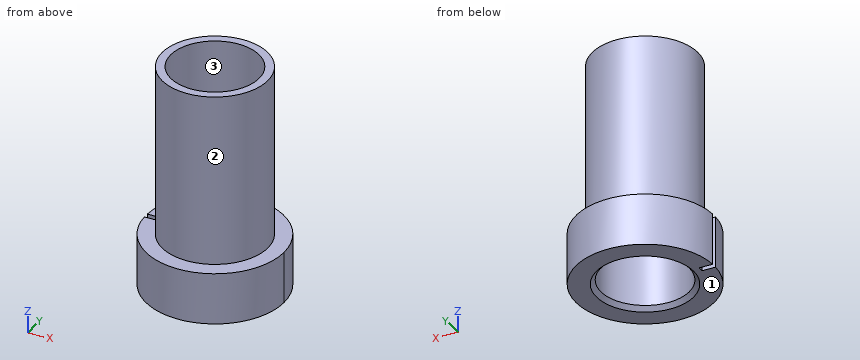
Autodesk Fusion 360 part; units mm, degrees
sketch "Sketch1" plane through (0, 0, 0) normal (0, 0, 1) x (1, 0, 0) in component "SpoolBottom"
  circle A0 centre (0, 0) radius 6.35
  dimension "d49" = 12.7
extrude "Extrude1" add sketch "Sketch1" along normal blind 4.7625 in component "SpoolBottom"
sketch "Sketch2" plane through (0, 0, 4.7625) normal (0, 0, 1) x (-1, 0, 0) in component "SpoolBottom"
  circle A0 centre (0, 0) radius 6.35
  circle A1 centre (0, 0) radius 4.8617
  dimension "d52" = 9.7234
extrude "Extrude2" add sketch "Sketch2" along normal blind 15.875 contours A1 in component "SpoolBottom"
sketch "Sketch3" plane through (0, 0, 20.6375) normal (0, 0, 1) x (-1, 0, 0) in component "SpoolBottom"
  circle A0 centre (0, 0) radius 4.8617
  circle A1 centre (0, 0) radius 4.068
  dimension "d55" = 8.1359
extrude "Extrude3" cut sketch "Sketch3" against normal blind 21.59 contours A1 in component "SpoolBottom"
chamfer "Chamfer1" distance 0.3969 angle 45 1 edges at (3.7927, 1.471, 0) in component "SpoolBottom"
sketch "Sketch4" plane through (0, 0, 4.7625) normal (0, 0, 1) x (-1, 0, 0) in component "SpoolBottom"
  circle A0 centre (0, 0) radius 4.8617
  circle A1 centre (0, 0) radius 6.35
  line L0 (5.0818, 0.2586) -> (6.5041, 0.2586)
  line L1 (6.5041, 0.2586) -> (6.5041, -0.2527)
  line L2 (6.5041, -0.2527) -> (5.0818, -0.2527)
  line L3 (5.0818, -0.2527) -> (5.0818, 0.2586)
extrude "Extrude4" cut sketch "Sketch4" against normal blind 4.826 contours A1 L0 L2 L3 picked at (5.5046, 0.002) in component "SpoolBottom"
component "SpoolBottom" placed x (1, 0, 0) y (0, 1, 0) z (0, 0, 1) at (0, 0, 0)
equation "d50 = ( 3 / 16 ) * 1 in"
equation "d52 = ( 5 / 16 ) * 1 in + ( 1 / 128 ) * 1 in + ( 2 / 32 ) * 1 in"
equation "d53 = ( 5 / 8 ) * 1 in"
equation "d55 = ( 5 / 16 ) * 1 in + ( 1 / 128 ) * 1 in"
equation "d58 = ( 1 / 64 ) * 1 in"
Source: CAD feature listing. Evaluate the final solid. Frame: model axes, mm. Face numbers are marked on the shaded views. Give positions to 0.01 mm unless a question says otherwise; leave off trailing zeros. Write each loop counter-clockwise with the first axis right and the second up, starting at its lowest first coordinate (ties: lowest second). Pieces come first, ordered by that corner, then holes.
1. Material intervals for line 1 along X through (y, z) = (0, 5); line 2 along Y through (x, z) = (0, 4.5), sorted ascending.
2. Pull-direction query (X, two-part tool) for the marked faces 1, 2 and 3; classes: +X half, -X half, draft (parallel to the pull), parting line (faces both ways), or undercut.
3. Section query A-A (x = 0). Return the cut outline in (y, z), then the cut area to 3 significant figures.
4. First-contact query: pin 1 (4 mm diameter, centred on x = 0.5, y = -0.5, fed in from +Z); pin 2 (4 mm diameter, centred on x = 3.5, z = 17.5, fed in from -Y); pin 3 (1 mm diameter, centred on x = -5.5, z = 3, fed in from -Y); pin 4 (1 mm diameter, centred on y = 3, z = 15.5, fed in from -X). Flat tips, straight axial feed; report the tip coordinate or a pass-through.
5. Section query B-B (z = 5). Return the cut outline in (x, y).
Output values:
1. line 1: x = -4.86 to -4.07, 4.07 to 4.86
1. line 2: y = -6.35 to -4.07, 4.07 to 6.35
2. face 1: draft
2. face 2: parting line
2. face 3: undercut
3. outline: (-6.35, 0) - (-4.46, 0) - (-4.07, 0.4) - (-4.07, 20.64) - (-4.86, 20.64) - (-4.86, 4.76) - (-6.35, 4.76) - close; (4.07, 0.4) - (4.46, 0) - (6.35, 0) - (6.35, 4.76) - (4.86, 4.76) - (4.86, 20.64) - (4.07, 20.64) - close
3. area: 46.8 mm2
4. pin 1: passes through
4. pin 2: stops at y = -4.62
4. pin 3: stops at y = -3.91
4. pin 4: stops at x = -4.17
5. outline: circle Ø9.72 at (0, 0); hole circle Ø8.14 at (0, 0)
